Read the model definition and answer for the solid it produces. Units are mm, in the model's axes. A direction names the side the tool comes from. Give positions to 0.01 mm unless a question says otherwise; leave off trailing zeros. Write each loop counter-clockwise with the first axis right and the second up, starting at its lowest first coordinate (ties: lowest second). Pieces come first, ordered by that corner, then holes. Notation, with made-up numbers: (47, -29.5) -> (77, -29.5) arc R25 cw to (77, -3.5) -> close; hole circle Ø10 at (-24.5, 5). An arc over 180 degrees is marked (long way). Put each result on its own line as item: value. Start each with the question number.
from build123d import *

# Parameters (mm, degrees)
F1_DEPTH = 5
F2_R     = 2
F3_R     = 1.5
F4_DEPTH = 5.001
F3_R_2   = 3.5
F5_DEPTH = 3
F7_DEPTH = 5


with BuildPart() as f1:
    # F0 (on Top) → F1 (new body)
    with BuildSketch(Plane.XY):
        Polygon((0, 15), (0, 0), (40, 0), (40, 20), (0, 20), (-25, 20), (-25, 0), (-5, 0), (-5, 5), (-20, 5), (-20, 15), align=None)
    extrude(amount=F1_DEPTH)

    # F2
    f2_edges = [f1.edges().sort_by_distance(p)[0] for p in [
        (-25, 0, 2.5),
        (-25, 20, 2.5),
        (40, 0, 2.5),
        (40, 20, 2.5),
        (0, 0, 2.5),
        (0, 15, 2.5),
        (-5, 0, 2.5),
        (-20, 5, 2.5),
        (-5, 5, 2.5),
        (-20, 15, 2.5),
    ]]
    fillet(f2_edges, radius=F2_R)

    # F3 (on face) → F4 (cut, through all)
    with BuildSketch(Plane.XY.offset(5)):
        with Locations((32.5, 10)):
            Circle(F3_R)
        with Locations((22.5, 10)):
            Circle(F3_R)
    extrude(amount=-F4_DEPTH, mode=Mode.SUBTRACT)

    # F3 (on face) → F5 (cut)
    with BuildSketch(Plane.XY.offset(5)):
        with Locations((22.5, 10)):
            Circle(F3_R_2)
        with Locations((22.5, 10)):
            Circle(F3_R, mode=Mode.SUBTRACT)
        with Locations((32.5, 10)):
            Circle(F3_R_2)
        with Locations((32.5, 10)):
            Circle(F3_R, mode=Mode.SUBTRACT)
    extrude(amount=-F5_DEPTH, mode=Mode.SUBTRACT)

    # F6 (on face) → F7 (cut, through all)
    with BuildSketch(Plane.XY.offset(5)):
        with BuildLine():
            ThreePointArc((26, 10), (22.5, 6.5), (19, 10))
            Line((19, 10), (19, 0))
            Line((19, 0), (26, 0))
            Line((26, 0), (26, 10))
        make_face()
    extrude(amount=-F7_DEPTH, mode=Mode.SUBTRACT)


solid = f1.part
1) Each of these flat-tipped pins is pushed along its axis until it touches: pin 1 Ø5 at (x, y) = (22.5, 10) entering from +Z; pin 2 Ø1 at (x, y) = (24, 2.5) entering from +Z. Where does it stop, or does it pass through?
2) For faces 1 (the face through (22, 8, 2)), 2 (the face through (7, 10, 5)), 3 (the face through (-0.57, 14.4, 2.54)), 4 (the face through (32, 8, 2)), 5 (the face through (-19.4, 5.57, 2.54)), determine the directions among +Z, -Z, +X, -X, +Y, -Y from which every point of the face is accessible in a straight line to the end or side of a thin tool.
3) A cutting plane is placed at A-A on z = 0.65. Give the vertices of the cut face in (x, y).
4) A cutting plane is placed at D-D on x = -12.5. Give the vertices of the cut face in (y, z).
5) A cutting plane is placed at C-C on z = 3.85. Give the vertices of the cut face in (x, y), and give its area (3 significant figures).
6) Straight lines are drawn through the part: line 1 (Y direction, x = 32.5, z = 1.55); line 2 (X direction, y = 9.75, z = 2.3); line 3 (X direction, y = 3.75, z = 3.2). For each, find the intervals that lie inside material, in ascending order. Write a range as [from, to].
7) For a pull along X with two mould halves and no side action, classify faces 6 (the face through (7, 10, 0)), 7 (the face through (-25, 10, 2)), 8 (the face through (34.115, 6.895, 3.521)) as pulls with the +X half, pulls with the -X half, needs draft (parallel to the pull), parting line crosses it, or undercut.
8) A cutting plane is placed at B-B on x = 22.5. Give the vertices of the cut face in (y, z).
Results found:
1. pin 1: stops at z = 2
1. pin 2: passes through
2. face 1: +Z, -Y
2. face 2: +Z, +X, -X, +Y, -Y
2. face 3: +Z, -Z, -Y
2. face 4: +Z
2. face 5: +Z, -Z
3. outline: (-25, 2) arc R2 ccw to (-23, 0) -> (-7, 0) arc R2 ccw to (-5, 2) -> (-5, 3) arc R2 ccw to (-7, 5) -> (-18, 5) arc R2 cw to (-20, 7) -> (-20, 13) arc R2 cw to (-18, 15) -> (-2, 15) arc R2 cw to (0, 13) -> (0, 2) arc R2 ccw to (2, 0) -> (19, 0) -> (19, 10) arc R3.5 ccw to (26, 10) -> (26, 0) -> (38, 0) arc R2 ccw to (40, 2) -> (40, 18) arc R2 ccw to (38, 20) -> (-23, 20) arc R2 ccw to (-25, 18) -> close; hole circle Ø3 at (22.5, 10); hole circle Ø3 at (32.5, 10)
4. outline: (0, 0) -> (5, 0) -> (5, 5) -> (0, 5) -> close; (15, 0) -> (20, 0) -> (20, 5) -> (15, 5) -> close
5. outline: (-25, 2) arc R2 ccw to (-23, 0) -> (-7, 0) arc R2 ccw to (-5, 2) -> (-5, 3) arc R2 ccw to (-7, 5) -> (-18, 5) arc R2 cw to (-20, 7) -> (-20, 13) arc R2 cw to (-18, 15) -> (-2, 15) arc R2 cw to (0, 13) -> (0, 2) arc R2 ccw to (2, 0) -> (19, 0) -> (19, 10) arc R3.5 cw to (26, 10) -> (26, 0) -> (38, 0) arc R2 ccw to (40, 2) -> (40, 18) arc R2 ccw to (38, 20) -> (-23, 20) arc R2 ccw to (-25, 18) -> close; hole circle Ø7 at (32.5, 10)
5. area: 944 mm²
6. line 1: y = [0, 8.5], [11.5, 20]
6. line 2: x = [-25, -20], [0, 19], [26, 29.01], [35.99, 40]
6. line 3: x = [-25, -5.15], [0, 19], [26, 40]
7. face 6: needs draft
7. face 7: pulls with the -X half
7. face 8: undercut
8. outline: (6.5, 0) -> (8.5, 0) -> (8.5, 2) -> (6.5, 2) -> close; (11.5, 0) -> (20, 0) -> (20, 5) -> (13.5, 5) -> (13.5, 2) -> (11.5, 2) -> close
